Job drawing, mm, ordinate dimensions from the low corner. One solid piece. A direction names the side the tool comes from. Give positions to 0.01 mm unless a question says otherwise; leave off trailing zeros. Order: outer loops, then holes, each group sorted by start corner. A loop starts at its lowest first (then second) coordinate and runs counter-clockwise, first axis right, second up. Notation, with made-up numbers: M 86.5,-27 L 106.5,-27 A24 ccw 106.5,9 Z; hole C 71.25,87.5 d2. An arc over 180 degrees is marked long. Use CSV: the item, a comma, the result in double quotes. Start each with the question number.
Item 1: Wall check: line 1 along X through (y, z) = (11.9, 50.34); line 2 along X through (y, z) = (11.8, 2.54); line 3 along Z through (x, y) = (2.54, 11.5). Give the ranges that are in metal, low to high.
Item 2: Band-saw the part on C-C on z = 50.34. Write the cut outline in (x, y), plus the area to 3 significant figures.
Item 3: Band-saw the part on B-B on z = 17.74. Write the cut outline in (x, y), plus the area to 3 significant figures.
Item 4: Band-saw the part on D-D on y = 3.25. Write the cut outline in (x, z).
Item 5: Which spindle directions (+Z, -Z, +X, -X, +Y, -Y) get a long thin tool onto all of the face, cutting with end or side? Do the marked faces 1, 2 and 3. Say none if no direction does.
Item 6: Band-saw the part on A-A on x = 2.54. Write the cut outline in (y, z), plus the area to 3 significant figures.
Item 7: Pin check, flat tips, straight feed: P1, Ø1.2, axis at y = 11.5, z = 33, coming from the +X side; P2, Ø4, axis at x = 2.54, z = 45.64, coming from the -Y side; P3, Ø2, axis at x = 62.5, y = 5.5, coming from the +Z side. Stop position of each tip, or through.
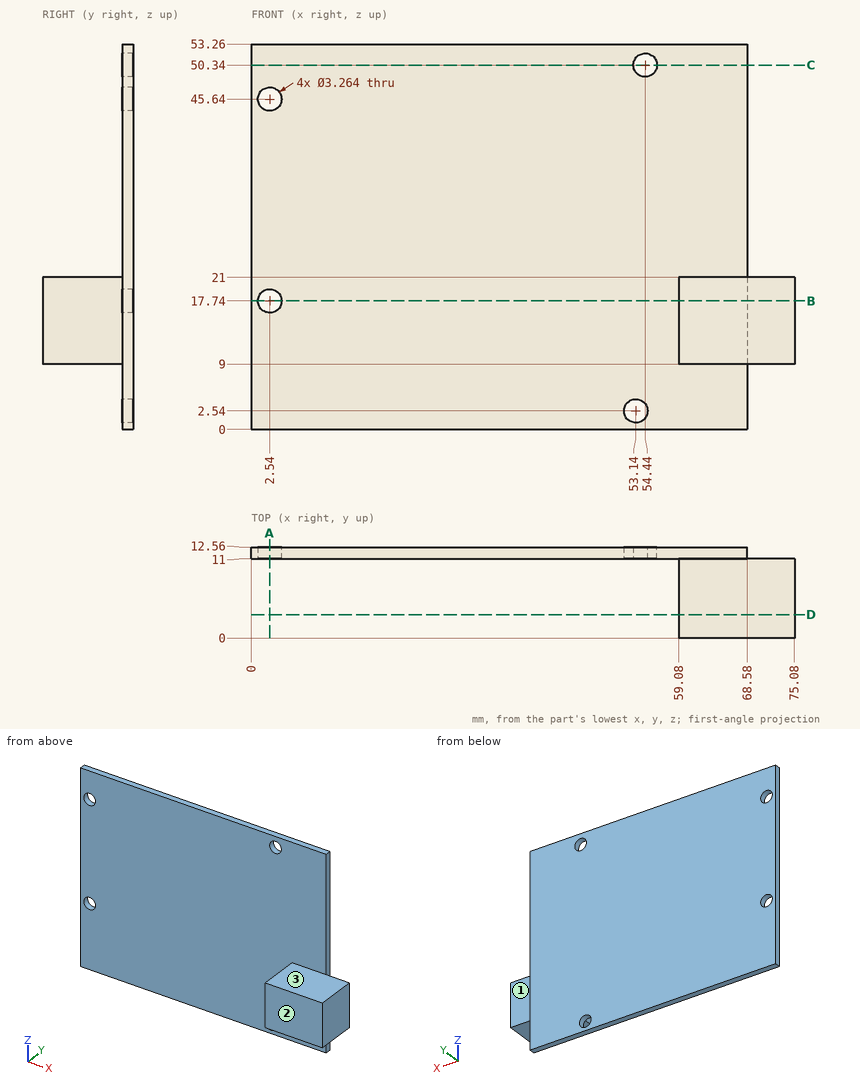
Model answer:
1,line 1,"x = 0 to 52.81, 56.07 to 68.58"
1,line 2,"x = 0 to 51.51, 54.77 to 68.58"
1,line 3,"z = 0 to 16.11, 19.37 to 44.01, 47.27 to 53.26"
2,outline,"M 0,11 L 52.81,11 L 52.81,12.56 L 0,12.56 Z; M 56.07,11 L 68.58,11 L 68.58,12.56 L 56.07,12.56 Z"
2,area,"102 mm^2"
3,outline,"M 0,11 L 0.91,11 L 0.91,12.56 L 0,12.56 Z; M 4.17,11 L 59.08,11 L 59.08,0 L 75.08,0 L 75.08,11 L 68.58,11 L 68.58,12.56 L 4.17,12.56 Z"
3,area,"278 mm^2"
4,outline,"M 59.08,9 L 75.08,9 L 75.08,21 L 59.08,21 Z"
5,face 1,"+Z, -Z, +X, +Y"
5,face 2,"+Z, -Z, +X, -X, -Y"
5,face 3,"+Z, +X, -X, -Y"
6,outline,"M 11,0 L 12.56,0 L 12.56,16.11 L 11,16.11 Z; M 11,19.37 L 12.56,19.37 L 12.56,44.01 L 11,44.01 Z; M 11,47.27 L 12.56,47.27 L 12.56,53.26 L 11,53.26 Z"
6,area,"72.9 mm^2"
7,P1,"stops at x = 68.58"
7,P2,"stops at y = 11"
7,P3,"stops at z = 21"
